Source: CAD feature listing. Evaluate the final solid. Frame: model axes, mm. A direction names the side the tool comes from. Round coordinates to 2 decimals unless told otherwise and drop trailing zeros. Write each loop counter-clockwise with the first axis right and the second up, starting at its lowest first coordinate (ties: lowest second). Pieces come first, ordered by that corner, then holes. Notation, with made-up numbers: (25.25, 52.25) -> (56.25, 52.25) arc R18 cw to (56.25, 63.25) -> close; hole circle Ø7 at (-38.5, 43). An arc over 180 degrees is marked (long way). Put each result on its own line as item: value.
```python
from build123d import *

# Parameters (mm, degrees)
SKETCH1_W                      = 110
SKETCH1_H                      = 89
SKETCH1_R                      = 4.75
BOSS_EXTRUDE1_DEPTH            = 10
SKETCH1_3_R                    = 4.75
SKETCH1_3_R_2                  = 1.75
BOSS_EXTRUDE2_DEPTH            = 15
SKETCH2_W                      = 110
SKETCH2_H                      = 36
CBORE_FOR_M3_SHCS1_D           = 3.4
CBORE_FOR_M3_SHCS1_CBORE_D     = 6.5
CBORE_FOR_M3_SHCS1_CBORE_DEPTH = 33


with BuildPart() as part:
    # Sketch1 → Boss-Extrude1 (new body)
    with BuildSketch(Plane.XY):
        Rectangle(SKETCH1_W, SKETCH1_H)
        with Locations((44.5, 29.5)):
            Circle(SKETCH1_R, mode=Mode.SUBTRACT)
        with Locations((44.5, -29.5)):
            Circle(SKETCH1_R, mode=Mode.SUBTRACT)
        with Locations((-44.5, -29.5)):
            Circle(SKETCH1_R, mode=Mode.SUBTRACT)
        with Locations((-44.5, 29.5)):
            Circle(SKETCH1_R, mode=Mode.SUBTRACT)
    extrude(amount=BOSS_EXTRUDE1_DEPTH)

    # Sketch1<3> → Boss-Extrude2 (add)
    with BuildSketch(Plane.XY):
        with Locations((-44.5, 29.5)):
            Circle(SKETCH1_3_R)
        with Locations((-44.5, 29.5)):
            Circle(SKETCH1_3_R_2, mode=Mode.SUBTRACT)
        with Locations((44.5, 29.5)):
            Circle(SKETCH1_3_R)
        with Locations((44.5, 29.5)):
            Circle(SKETCH1_3_R_2, mode=Mode.SUBTRACT)
        with Locations((44.5, -29.5)):
            Circle(SKETCH1_3_R)
        with Locations((44.5, -29.5)):
            Circle(SKETCH1_3_R_2, mode=Mode.SUBTRACT)
        with Locations((-44.5, -29.5)):
            Circle(SKETCH1_3_R)
        with Locations((-44.5, -29.5)):
            Circle(SKETCH1_3_R_2, mode=Mode.SUBTRACT)
    extrude(amount=BOSS_EXTRUDE2_DEPTH)

    # Sketch2 → section 1 of loft1
    with BuildSketch(Plane(origin=(0, -82, 0), x_dir=(1, 0, 0), z_dir=(0, 1, 0)), mode=Mode.PRIVATE) as loft1_s1:
        with Locations((0, -5)):
            Rectangle(SKETCH2_W, SKETCH2_H)
    # loft from a face of the part (loft1)
    loft([part.faces().sort_by_distance((0, -44.5, 5))[0], loft1_s1.sketch])

    # CBORE for M3 SHCS1 (through all)
    with Locations(Plane(origin=(0, -44.5, 0), x_dir=(1, 0, 0), z_dir=(0, 1, 0))):
        with Locations((-25, 7), (25, 7), (25, -17), (-25, -17)):
            CounterBoreHole(CBORE_FOR_M3_SHCS1_D / 2, CBORE_FOR_M3_SHCS1_CBORE_D / 2, CBORE_FOR_M3_SHCS1_CBORE_DEPTH)


solid = part.part
```
Q1. Material intervals for line 1 (X direction, y = -80, z = -7); line 2 (X direction, y = -66, z = 17); line 3 (Z direction, x = 25, y = -80.5), sorted ascending. Write a range as [from, to].
Ans:
line 1: x = [-55, -26.7], [-23.3, 23.3], [26.7, 55]
line 2: x = [-55, -28.25], [-21.75, 21.75], [28.25, 55]
line 3: z = [-12.48, -8.7], [-5.3, 15.3], [18.7, 22.48]
Q2. Cut plane C-C on z = -7. Output: boundary loops of the cut face in (x, y).
Ans:
outline: (-55, -82) -> (-26.7, -82) -> (-26.7, -77.5) -> (-28.25, -77.5) -> (-28.25, -64.69) -> (-55, -64.69) -> close; (-23.3, -82) -> (23.3, -82) -> (23.3, -77.5) -> (21.75, -77.5) -> (21.75, -64.69) -> (-21.75, -64.69) -> (-21.75, -77.5) -> (-23.3, -77.5) -> close; (26.7, -82) -> (55, -82) -> (55, -64.69) -> (28.25, -64.69) -> (28.25, -77.5) -> (26.7, -77.5) -> close
Q3. Cut plane B-B on y = -29.5. Output: boundary loops of the cut face in (x, z), and give its area (3 significant figures).
Ans:
outline: (-55, 0) -> (-46.25, 0) -> (-46.25, 15) -> (-49.25, 15) -> (-49.25, 10) -> (-55, 10) -> close; (-42.75, 0) -> (42.75, 0) -> (42.75, 15) -> (39.75, 15) -> (39.75, 10) -> (-39.75, 10) -> (-39.75, 15) -> (-42.75, 15) -> close; (46.25, 0) -> (55, 0) -> (55, 10) -> (49.25, 10) -> (49.25, 15) -> (46.25, 15) -> close
area: 1,090 mm^2
Q4. Pin query (flat end, axial travel): pin 1 (7.5 mm diameter, centred on x = 42.5, y = 30, fed in from +Z); pin 2 (3 mm diameter, centred on x = 25.5, z = 18.5, fed in from +Y); pin 3 (2 mm diameter, centred on x = 29.5, y = -61, fed in from -Z); pin 4 (2 mm diameter, centred on x = 25, z = -7, fed in from +Y). Return the tip coordinate at first contact, or that it passes through.
Ans:
pin 1: stops at z = 15
pin 2: stops at y = -77.5
pin 3: stops at z = -6.07
pin 4: passes through
Q5. Draft query along Z for faces 1 (the flat face through (-55, -34, 5)), 2 (the cylindrical face through (-26.57, -79.78, 17.65)), 3 (the flat face through (-42, -29, 15)), 4 (the flat face through (0.77, -63.51, -6.59)). Return one class per face: +Z half, -Z half, draft (parallel to the pull), parting line (faces both ways), or undercut.
Ans:
face 1: draft
face 2: undercut
face 3: +Z half
face 4: -Z half
Q6. Reachability of faces 5 (the cylindrical face through (-25.423, -68.629, 13.778)), 6 (the cylindrical face through (-42.883, 28.83, 7.395)), 7 (the cylindrical face through (-48.27, 26.61, 12.46)), 8 (the cylindrical face through (23.43, -79.78, 17.65)), 9 (the flat face through (47, -29, 15)) from +Z, -Z, +X, -X, +Y, -Y: full face, straight path, thin tool, end or side. Return the list, or none.
Ans:
face 5: +Y
face 6: +Z, -Z
face 7: +Z
face 8: +Y, -Y
face 9: +Z, +X, -X, +Y
Q7. Cut plane D-D on x = 12. Output: boundary loops of the cut face in (y, z).
Ans:
outline: (-82, -13) -> (-44.5, 0) -> (44.5, 0) -> (44.5, 10) -> (-44.5, 10) -> (-82, 23) -> close
Q8. Cut plane A-A on x = 44.5. Output: boundary loops of the cut face in (y, z), and give its area (3 significant figures).
Ans:
outline: (-82, -13) -> (-44.5, 0) -> (-31.25, 0) -> (-31.25, 15) -> (-34.25, 15) -> (-34.25, 10) -> (-44.5, 10) -> (-82, 23) -> close; (-27.75, 0) -> (27.75, 0) -> (27.75, 15) -> (24.75, 15) -> (24.75, 10) -> (-24.75, 10) -> (-24.75, 15) -> (-27.75, 15) -> close; (31.25, 0) -> (44.5, 0) -> (44.5, 10) -> (34.25, 10) -> (34.25, 15) -> (31.25, 15) -> close
area: 1,740 mm^2
